```python
from build123d import *

# Parameters (mm, degrees)
SKETCH1_R           = 5
SKETCH1_R_2         = 4.7625
BOSS_EXTRUDE1_DEPTH = 6.35


with BuildPart() as part:
    # Sketch1 → Boss-Extrude1 (new body)
    with BuildSketch(Plane(origin=(0, 0, 0), x_dir=(1, 0, 0), z_dir=(0, 1, 0))):
        with BuildLine():
            Line((10, 40), (10, 0))
            ThreePointArc((10, 0), (7.5, -6.614378278), (1.25, -9.921567416))
            Line((1.25, -9.921567416), (-57.8125, -17.362742979))
            ThreePointArc((-57.8125, -17.362742979), (-76.694591069, -5.247916638), (-68.140184424, 15.491526637))
            Line((-68.140184424, 15.491526637), (-4.651533957, 48.852300935))
            ThreePointArc((-4.651533957, 48.852300935), (5.171298697, 48.559069446), (10, 40))
        make_face()
        with Locations(Location((0, 0, 0), (0, 0, 270))):
            Circle(SKETCH1_R, mode=Mode.SUBTRACT)
        with Locations(Location((0, 40, 0), (0, 0, 270))):
            Circle(SKETCH1_R, mode=Mode.SUBTRACT)
        with Locations(Location((-60, 0, 0), (0, 0, 270))):
            Circle(SKETCH1_R_2, mode=Mode.SUBTRACT)
    extrude(amount=-BOSS_EXTRUDE1_DEPTH)


solid = part.part
```
Read the model definition and answer for the solid it produces. Units are mm, in the model's axes. Coordinates: 2 decimals unless noted, no trailing zeros. Write each loop counter-clockwise with the first axis right and the second up, starting at its lowest first coordinate (ties: lowest second). Pieces come first, ordered by that corner, then holes. Notation, with made-up numbers: (55, 88) -> (66, 88) arc R10 ccw to (66, 95) -> close; hole circle Ø6 at (2, -28.5). An arc over 180 degrees is marked (long way). Answer as a JSON object with one key per item and string values.
Q1. Consider line 1 (X direction, y = -3, z = 0); line 2 (Z direction, x = 1.5, y = -4.5); line 3 (Z direction, x = -58, y = -6). Determine where each line is inside the solid, lowest interval first. Write a range as [from, to].
The answers:
{"line 1": "x = [-77.5, -64.76], [-55.24, -5], [5, 10]", "line 2": "z = [-49.89, -44.77], [-35.23, -4.77], [4.77, 9.89]", "line 3": "z = [-20.82, -4.32], [4.32, 17.39]"}
Q2. The part is cut by section D-D on x = -60. Give the vertices of the cut face in (y, z).
The answers:
{"outline": "(-6.35, -19.77) -> (0, -19.77) -> (0, -4.76) -> (-6.35, -4.76) -> close; (-6.35, 4.76) -> (0, 4.76) -> (0, 17.5) -> (-6.35, 17.5) -> close"}
Q3. Determine the mould class of faces 1 (the cylindrical face through (5.05, -3.13, -48.63)), 2 (the flat face through (-23, 0, -9)), 3 (the cylindrical face through (-55.28, -3.13, -0.62)) for opening direction X: pulls with the +X half, pulls with the -X half, needs draft (parallel to the pull), parting line crosses it, or undercut.
The answers:
{"face 1": "parting line crosses it", "face 2": "needs draft", "face 3": "undercut"}
Q4. Flat-ended cylindrical pins translate along their axes: pin 1 Ø7.5 at (x, z) = (-60, 0) entering from -Y; pin 2 Ø1 at (x, y) = (-5.5, -2) entering from +Z (3 decimals); pin 3 Ø2 at (y, z) = (-4.5, 9) entering from +X; pin 4 Ø1.5 at (y, z) = (-1, -24.5) entering from -X. Find the tip coordinate at first contact, or state that the pin passes through.
The answers:
{"pin 1": "passes through", "pin 2": "stops at z = 10.835", "pin 3": "stops at x = 6", "pin 4": "stops at x = -52.42"}
Q5. The part is cut by section C-C on x = 0. Give the vertices of the cut face in (y, z).
The answers:
{"outline": "(-6.35, -50) -> (0, -50) -> (0, -45) -> (-6.35, -45) -> close; (-6.35, -35) -> (0, -35) -> (0, -5) -> (-6.35, -5) -> close; (-6.35, 5) -> (0, 5) -> (0, 10.08) -> (-6.35, 10.08) -> close"}
Q6. The part is cut by section A-A on y = -2.75. Give the number of separate pieces and of enclosed holes in the cut face, then the cut area to 3 significant figures.
The answers:
{"separate pieces": "1", "enclosed holes": "3", "area": "3,780 mm2"}
Q7. The part is cut by section B-B on z = 1. Give the vertices of the cut face in (x, y), then the cut area to 3 significant figures.
The answers:
{"outline": "(-77.47, -6.35) -> (-64.66, -6.35) -> (-64.66, 0) -> (-77.47, 0) -> close; (-55.34, -6.35) -> (-4.9, -6.35) -> (-4.9, 0) -> (-55.34, 0) -> close; (4.9, -6.35) -> (9.95, -6.35) -> (9.95, 0) -> (4.9, 0) -> close", "area": "434 mm2"}
